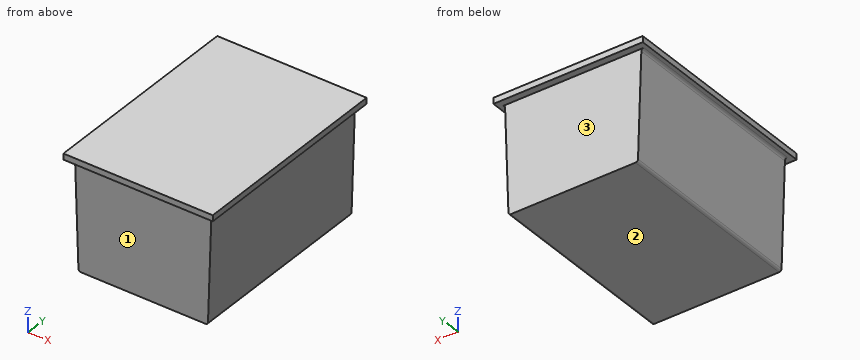
```python
from build123d import *

# Parameters (mm, degrees)
F1_DEPTH = 420
F3_DEPTH = 14


# Not quite as in the source:
# - a pattern or mirror of a feature is missing from the dataset's text; its kind, count and spacing are read off the source's solid


with BuildPart() as f1:
    # F0 (on Front) → F1 (new body)
    with BuildSketch(Plane.XZ):
        with BuildLine():
            Line((150, 0), (0, 0))
            Line((0, 0), (-150, 0))
            Line((-150, 0), (-150, -12))
            Line((-150, -12), (-141.8420265222, -12))
            ThreePointArc((-141.8420265222, -12), (-138.3636891874, -13.4081802125), (-136.8446021756, -16.8395322458))
            Line((-136.8446021756, -16.8395322458), (-130.1553978244, -225.1604677542))
            ThreePointArc((-130.1553978244, -225.1604677542), (-128.6363108126, -228.5918197875), (-125.1579734778, -230))
            Line((-125.1579734778, -230), (0, -230))
            Line((0, -230), (125.1579734778, -230))
            ThreePointArc((125.1579734778, -230), (128.6363108126, -228.5918197875), (130.1553978244, -225.1604677542))
            Line((130.1553978244, -225.1604677542), (136.8446021756, -16.8395322458))
            ThreePointArc((136.8446021756, -16.8395322458), (138.3636891874, -13.4081802125), (141.8420265222, -12))
            Line((141.8420265222, -12), (150, -12))
            Line((150, -12), (150, 0))
        make_face()
    extrude(amount=F1_DEPTH)

    # F2 (on face) → F3 (cut)
    with BuildSketch(Plane.XZ.offset(420)):
        with BuildLine():
            Line((141.8420265222, -12), (-141.8420265222, -12))
            ThreePointArc((-141.8420265222, -12), (-138.3636891874, -13.4081802125), (-136.8446021756, -16.8395322458))
            Line((-136.8446021756, -16.8395322458), (-130.1553978244, -225.1604677542))
            ThreePointArc((-130.1553978244, -225.1604677542), (-128.6363108126, -228.5918197875), (-125.1579734778, -230))
            Line((-125.1579734778, -230), (125.1579734778, -230))
            ThreePointArc((125.1579734778, -230), (128.6363108126, -228.5918197875), (130.1553978244, -225.1604677542))
            Line((130.1553978244, -225.1604677542), (136.8446021756, -16.8395322458))
            ThreePointArc((136.8446021756, -16.8395322458), (138.3636891874, -13.4081802125), (141.8420265222, -12))
        make_face()
    f3 = extrude(amount=-F3_DEPTH, mode=Mode.SUBTRACT)

    # F3_copies: F3 across plane
    add(f3.mirror(Plane.ZX.offset(-210)), mode=Mode.SUBTRACT)


solid = f1.part
```
For this review, take the finished solid that the model builds, in its own axes (mm). Face numbers are marked on the shaded views. A direction names the side the tool comes from. Round coordinates to 2 decimals unless told otherwise and drop trailing zeros. Write each loop counter-clockwise with the first axis right and the second up, starting at its lowest first coordinate (ties: lowest second). Pieces come first, ordered by that corner, then holes. Notation, with made-up numbers: (-32, 31.25) - (-28, 31.25) arc R16 cw to (-28, 35.25) - close; hole circle Ø2 at (76, 78). An arc over 180 degrees is marked (long way). Put each result on its own line as item: value.
Q1. Insertion check: pin 1 Ø8 at (x, z) = (99, -55.5) entering from +Y; pin 2 Ø1.5 at (x, z) = (-54, -108.5) entering from -Y; pin 3 Ø3 at (y, z) = (-285.5, -39) entering from -X. Each pin has a flat end and moves straight along its axis. Give the tip position at first contact, or say it passes through.
Solved:
pin 1: stops at y = -14
pin 2: stops at y = -406
pin 3: stops at x = -136.18
Q2. We need section B-B (y = -147). Give the boundary of the cut face in (x, z), and give its area (3 significant figures).
Solved:
outline: (-150, -12) - (-141.84, -12) arc R5 cw to (-136.84, -16.84) - (-130.16, -225.16) arc R5 ccw to (-125.16, -230) - (125.16, -230) arc R5 ccw to (130.16, -225.16) - (136.84, -16.84) arc R5 cw to (141.84, -12) - (150, -12) - (150, 0) - (-150, 0) - close
area: 61,800 mm2
Q3. We need section C-C (z = -118.5). Give the boundary of the cut face in (x, y), and give its area (3 significant figures).
Solved:
outline: (-133.58, -406) - (133.58, -406) - (133.58, -14) - (-133.58, -14) - close
area: 105,000 mm2
Q4. We need section D-D (z = -45). Give the boundary of the cut face in (x, y).
Solved:
outline: (-135.94, -406) - (135.94, -406) - (135.94, -14) - (-135.94, -14) - close
Q5. Wall thickness on probe 1 along Y at (x, z) = (38, -140); probe 2 along X at (y, z) = (-255.5, -18); probe 3 along X at (y, z) = (-186.5, -107): over which ranges is each line inside the solid? List them lowest first.
Solved:
probe 1: y = -406 to -14
probe 2: x = -136.81 to 136.81
probe 3: x = -133.95 to 133.95
Q6. We need section A-A (x = 70.5). Give the boundary of the cut face in (y, z), and give its area (3 significant figures).
Solved:
outline: (-420, -12) - (-406, -12) - (-406, -230) - (-14, -230) - (-14, -12) - (0, -12) - (0, 0) - (-420, 0) - close
area: 90,500 mm2
Q7. Machinability: for the marked faces 1, 2 and 3, which of the approach directions +Z, -Z, +X, -X, +Y, -Y give a long, thin tool a straight path to every point of the face, cutting with its end or side? Answer none if there is none.
Solved:
face 1: -Z, +X, -X, -Y
face 2: -Z, +X, -X, +Y, -Y
face 3: -Z, +X, -X, +Y
